Input: part model. Units: mm. Frame: model coordinates. A direction names the side the tool comes from. Round coordinates to 2 decimals unless told otherwise and drop trailing zeros. Order: outer loops, then holes, each group sorted by start corner. A loop starts at its lowest first (then second) coordinate and runs counter-clockwise, first axis right, second up.
Item 1: Reachability of faces 1 (the flat face through (-22, -5, 12)), 2 (the flat face through (-51, -4, 19)), 3 (the flat face through (-38, -5, 1.5)), 4 (the flat face through (-43, -17.096, 10)) from +Z, -Z, +X, -X, +Y, -Y: full face, straight path, thin tool, end or side. Return the list, or none.
Item 2: Cut plane C-C on z = 9. Output: boundary loops of the cut face in (x, y), then the cut area to 3 significant figures.
Item 3: Cut plane D-D on y = 0.75. Output: boundary loops of the cut face in (x, z), then the cut area to 4 significant figures.
Item 4: Cut plane A-A on y = -6.25. Output: boundary loops of the cut face in (x, z).
Item 5: Mould query, pull axis X, two halves, no side actions, for faces 5 (the flat face through (-65.029, -5, 18)), 6 (the flat face through (-38, 1.604, 10)), 7 (the flat face through (-43, 7.904, 10)), 8 (the flat face through (-49.929, -5, 10)). Classes: released by +X, released by -X, zero draft, split by the parting line, or undercut.
Item 6: Line query: L1, parallel to Z at x = -23, y = -8.25; L2, parallel to Y at x = -41.5, z = 15; L3, parallel to X at y = 1.5, z = 16. Output: solid intervals per line, ascending.
Item 7: First-contact query: pin 1 (2 mm diameter, centred on x = -41.5, y = -6, fed in from +Z); pin 2 (1.8 mm diameter, centred on x = -52, y = -5, fed in from +Z); pin 3 (2 mm diameter, centred on x = -52.43, y = -4.6, fed in from +Z). Flat tips, straight axial feed; report the tip coordinate or a pass-through.
Item 8: Cut plane B-B on x = -25.5. Output: boundary loops of the cut face in (y, z), then the cut area to 3 significant figures.
```python
from build123d import *

# Parameters (mm, degrees)
SKETCH_1_W          = 45
SKETCH_1_H          = 25
EXTRUDE_2_DEPTH     = 19
SKETCH_4_W          = 23.6
SKETCH_4_H          = 12.4
CUT_EXTRUDE_2_DEPTH = 17.5
SKETCH_5_W          = 8
SKETCH_5_H          = 9
CUT_EXTRUDE_4_DEPTH = 7
SKETCH_6_R          = 1.1
CUT_EXTRUDE_6_DEPTH = 7.5
SKETCH_8_W          = 2.6
SKETCH_8_H          = 25
EXTRUDE_3_DEPTH     = 17.5


with BuildPart() as part:
    # 草圖1 → 填料-伸長2 (new body)
    with BuildSketch(Plane.XY):
        with Locations((-42.528991691, -4.596431101)):
            Rectangle(SKETCH_1_W, SKETCH_1_H)
    extrude(amount=EXTRUDE_2_DEPTH)

    # 草圖4 → 除料-伸長2 (cut)
    with BuildSketch(Plane.XY.offset(19)):
        with Locations((-38.128991691, -4.596431101)):
            Rectangle(SKETCH_4_W, SKETCH_4_H)
    extrude(amount=-CUT_EXTRUDE_2_DEPTH, mode=Mode.SUBTRACT)

    # 草圖5 → 除料-伸長4 (cut)
    with BuildSketch(Plane(origin=(-20.028991691, 0, 0), x_dir=(0, 0, -1), z_dir=(1, 0, 0))):
        with Locations((-8, -4.596431101)):
            Rectangle(SKETCH_5_W, SKETCH_5_H)
    extrude(amount=-CUT_EXTRUDE_4_DEPTH, mode=Mode.SUBTRACT)

    # 草圖6 → 除料-伸長6 (cut)
    with BuildSketch(Plane.XY.offset(19)):
        with Locations((-23.828991691, -4.596431101)):
            Circle(SKETCH_6_R)
        with Locations((-52.428991691, -4.596431101)):
            Circle(SKETCH_6_R)
    extrude(amount=-CUT_EXTRUDE_6_DEPTH, mode=Mode.SUBTRACT)

    # 草圖8 → 填料-伸長3 (add)
    with BuildSketch(Plane.XY.offset(19)):
        with Locations((-63.728991691, -4.596431101)):
            Rectangle(SKETCH_8_W, SKETCH_8_H)
    extrude(amount=EXTRUDE_3_DEPTH)


solid = part.part
```
From the geometry:
1. face 1: +X
1. face 2: +Z, +X, +Y, -Y
1. face 3: +Z
1. face 4: +Z, -Z, +X, -X, -Y
2. outline: (-65.03, -17.1) - (-20.03, -17.1) - (-20.03, -9.1) - (-26.33, -9.1) - (-26.33, -10.8) - (-49.93, -10.8) - (-49.93, 1.6) - (-26.33, 1.6) - (-26.33, -0.1) - (-20.03, -0.1) - (-20.03, 7.9) - (-65.03, 7.9) - close
2. area: 776 mm2
3. outline: (-65.03, 0) - (-20.03, 0) - (-20.03, 19) - (-26.33, 19) - (-26.33, 1.5) - (-49.93, 1.5) - (-49.93, 19) - (-62.43, 19) - (-62.43, 36.5) - (-65.03, 36.5) - close
3. area: 487.5 mm2
4. outline: (-65.03, 0) - (-20.03, 0) - (-20.03, 4) - (-26.33, 4) - (-26.33, 1.5) - (-49.93, 1.5) - (-49.93, 19) - (-62.43, 19) - (-62.43, 36.5) - (-65.03, 36.5) - close; (-26.33, 12) - (-20.03, 12) - (-20.03, 19) - (-26.33, 19) - close
5. face 5: released by -X
5. face 6: undercut
5. face 7: zero draft
5. face 8: undercut
6. L1: z = 0 to 4, 12 to 19
6. L2: y = -17.1 to -10.8, 1.6 to 7.9
6. L3: x = -65.03 to -49.93, -26.33 to -20.03
7. pin 1: stops at z = 1.5
7. pin 2: stops at z = 19
7. pin 3: stops at z = 11.5
8. outline: (-17.1, 0) - (7.9, 0) - (7.9, 19) - (-17.1, 19) - close; hole (-9.1, 4) - (-0.1, 4) - (-0.1, 12) - (-9.1, 12) - close
8. area: 403 mm2
